The listing builds one solid part. Answer for the finished solid, in the listing's coordinates (mm). Face numbers are marked on the shaded views. A direction names the side the tool comes from. Give positions to 0.01 mm unless a question says otherwise; leave off trailing zeros. Loops run counter-clockwise (first coordinate to the right, second up) from the corner with the lowest first, then second, coordinate; pieces in that order, holes last.
Item 1: Section A-A, the plane x = -65 is taken. Give the vertices of the cut face in (y, z).
Item 2: Consider line 1 along X through (y, z) = (2.5, 1.5); line 2 along Y through (x, z) = (65, 10.75); line 3 along X through (y, z) = (56, 13.5). Determine where each line is inside the solid, lowest interval first.
Item 3: A tool of negligible diameter and unlimited length cuts with its end or side. For the marked faces 1, 2, 3 and 4, from which of +Z, -Z, +X, -X, +Y, -Y can it reach the whole face along a straight path? Write none if from no direction.
Item 4: Section D-D, the plane y = -54 is taken. Give the vertices of the cut face in (x, z).
Item 5: Section C-C, the plane z = 16.25 is taken. Give the number of separate pieces and of enclosed holes in the cut face, and give its area (3 significant figures).
Item 6: Each of these flat-tipped pins is pushed along its axis until it touches: pin 1 Ø6 at (y, z) = (53.5, 9.5) entering from -X; pin 2 Ø2 at (y, z) = (70, 17) entering from +X; pin 3 Ø2 at (x, z) = (-25.5, 6) entering from +Y. Where does it stop, or does it pass through?
from build123d import *

# Parameters (mm, degrees)
F0_R     = 3.5
F1_DEPTH = 20
F2_R     = 20


with BuildPart() as f1:
    # F0 (on Top) → F1 (new body)
    with BuildSketch(Plane.XY):
        with BuildLine():
            Line((68.9, 27.5), (27.5, 27.5))
            Line((27.5, 27.5), (27.5, 68.9))
            ThreePointArc((27.5, 68.9), (21.642136, 83.042136), (7.5, 88.9))
            Line((7.5, 88.9), (-7.5, 88.9))
            ThreePointArc((-7.5, 88.9), (-21.642136, 83.042136), (-27.5, 68.9))
            Line((-27.5, 68.9), (-27.5, 27.5))
            Line((-27.5, 27.5), (-68.9, 27.5))
            ThreePointArc((-68.9, 27.5), (-83.042136, 21.642136), (-88.9, 7.5))
            Line((-88.9, 7.5), (-88.9, -7.5))
            ThreePointArc((-88.9, -7.5), (-83.042136, -21.642136), (-68.9, -27.5))
            Line((-68.9, -27.5), (-27.5, -27.5))
            Line((-27.5, -27.5), (-27.5, -68.9))
            ThreePointArc((-27.5, -68.9), (-21.642136, -83.042136), (-7.5, -88.9))
            Line((-7.5, -88.9), (7.5, -88.9))
            ThreePointArc((7.5, -88.9), (21.642136, -83.042136), (27.5, -68.9))
            Line((27.5, -68.9), (27.5, -27.5))
            Line((27.5, -27.5), (68.9, -27.5))
            ThreePointArc((68.9, -27.5), (83.042136, -21.642136), (88.9, -7.5))
            Line((88.9, -7.5), (88.9, 7.5))
            ThreePointArc((88.9, 7.5), (83.042136, 21.642136), (68.9, 27.5))
        make_face()
        with Locations((0, -65)):
            Circle(F0_R, mode=Mode.SUBTRACT)
        with Locations((0, -23)):
            Circle(F0_R, mode=Mode.SUBTRACT)
        with Locations((-65, 0)):
            Circle(F0_R, mode=Mode.SUBTRACT)
        with Locations((-23, 0)):
            Circle(F0_R, mode=Mode.SUBTRACT)
        with BuildLine():
            ThreePointArc((4, 0), (2.828427, -2.828427), (0, -4))
            ThreePointArc((0, -4), (-2.828427, -2.828427), (-4, 0))
            ThreePointArc((-4, 0), (-2.828427, 2.828427), (0, 4))
            ThreePointArc((0, 4), (2.828427, 2.828427), (4, 0))
        make_face(mode=Mode.SUBTRACT)
        with Locations((23, 0)):
            Circle(F0_R, mode=Mode.SUBTRACT)
        with Locations((0, 23)):
            Circle(F0_R, mode=Mode.SUBTRACT)
        with Locations((65, 0)):
            Circle(F0_R, mode=Mode.SUBTRACT)
        with Locations((0, 65)):
            Circle(F0_R, mode=Mode.SUBTRACT)
    extrude(amount=F1_DEPTH)

    # F2
    f2_edges = [f1.edges().sort_by_distance(p)[0] for p in [
        (27.5, 27.5, 10),
        (27.5, -27.5, 10),
        (-27.5, -27.5, 10),
        (-27.5, 27.5, 10),
    ]]
    fillet(f2_edges, radius=F2_R)


solid = f1.part
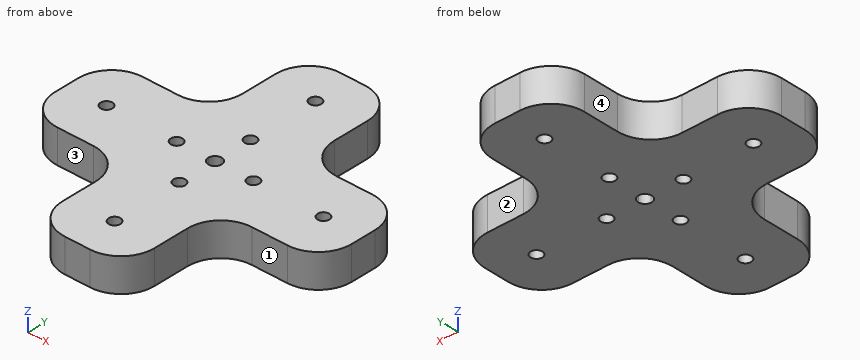
Worked answers:
1. outline: (-27.5, 0) - (-3.5, 0) - (-3.5, 20) - (-27.5, 20) - close; (3.5, 0) - (27.5, 0) - (27.5, 20) - (3.5, 20) - close
2. line 1: x = -88.9 to -67.45, -62.55 to -25.45, -20.55 to -3.12, 3.12 to 20.55, 25.45 to 62.55, 67.45 to 88.9
2. line 2: y = -27.5 to -3.5, 3.5 to 27.5
2. line 3: x = -27.5 to 27.5
3. face 1: +Z, -Z, +X, -Y
3. face 2: +Z, -Z, +X, +Y
3. face 3: +Z, -Z, -X, -Y
3. face 4: +Z, -Z, -X, +Y
4. outline: (-27.5, 0) - (27.5, 0) - (27.5, 20) - (-27.5, 20) - close
5. separate pieces: 1
5. enclosed holes: 9
5. area: 15,800 mm2
6. pin 1: stops at x = -27.5
6. pin 2: stops at x = 27.5
6. pin 3: stops at y = 79.44
